from build123d import *

# Parameters (mm, degrees)
SKETCH1_R           = 4.9609375
BOSS_EXTRUDE1_DEPTH = 75.692
SKETCH3_R           = 1.6256
CUT_EXTRUDE1_DEPTH  = 11.914472708
SKETCH3_3_R         = 2.511415146
SKETCH3_3_R_2       = 1.6256
BOSS_EXTRUDE2_DEPTH = 5.08
SKETCH4_R           = 1.580559699
SKETCH4_R_2         = 1.615968851
SKETCH4_R_3         = 1.651
CUT_EXTRUDE2_DEPTH  = 11.914472708
BOSS_EXTRUDE3_DEPTH = 5.500116
SKETCH6_R           = 1.5875
CUT_EXTRUDE3_DEPTH  = 17.414588708


with BuildPart() as part:
    # Sketch1 → Boss-Extrude1 (new body, symmetric)
    with BuildSketch(Plane(origin=(0, 0, 0), x_dir=(1, 0, 0), z_dir=(0, 1, 0))):
        with BuildLine():
            ThreePointArc((-54.898232946, 10.914472708), (-55.979756859, 9.486084273), (-57.024125462, 8.030308975))
            ThreePointArc((-57.024125462, 8.030308975), (-55.271492218, -9.123122127), (-40.64, 0))
            Line((-40.64, 0), (40.64, 0))
            ThreePointArc((40.64, 0), (55.271492218, -9.123122127), (57.024125462, 8.030308975))
            ThreePointArc((57.024125462, 8.030308975), (55.979756859, 9.486084273), (54.898232946, 10.914472708))
            Line((54.898232946, 10.914472708), (-54.898232946, 10.914472708))
        make_face()
        with Locations((-50.8, 0)):
            Circle(SKETCH1_R, mode=Mode.SUBTRACT)
        with Locations((50.8, 0)):
            Circle(SKETCH1_R, mode=Mode.SUBTRACT)
    extrude(amount=BOSS_EXTRUDE1_DEPTH, both=True)

    # Sketch3 → Cut-Extrude1 (cut, through all)
    with BuildSketch(Plane.XY):
        with Locations((-14.08707582, 68.405041605)):
            Circle(SKETCH3_R)
        with Locations((-26.78707582, 43.005041605)):
            Circle(SKETCH3_R)
    extrude(amount=-CUT_EXTRUDE1_DEPTH, mode=Mode.SUBTRACT)

    # Sketch3_3 → Boss-Extrude2 (add)
    with BuildSketch(Plane.XY):
        with Locations((-14.08707582, 68.405041605)):
            Circle(SKETCH3_3_R)
        with Locations((-14.08707582, 68.405041605)):
            Circle(SKETCH3_3_R_2, mode=Mode.SUBTRACT)
        with Locations((-26.78707582, 43.005041605)):
            Circle(SKETCH3_3_R)
        with Locations((-26.78707582, 43.005041605)):
            Circle(SKETCH3_3_R_2, mode=Mode.SUBTRACT)
    extrude(amount=BOSS_EXTRUDE2_DEPTH)

    # Sketch4 → Cut-Extrude2 (cut, through all)
    with BuildSketch(Plane.XY):
        with Locations((5.097142458, 69.338036856)):
            Circle(SKETCH4_R)
        with Locations((27.569466172, 69.326708036)):
            Circle(SKETCH4_R_2)
        with Locations((4.630258258, 15.178805596)):
            Circle(SKETCH4_R_3)
        with Locations((31.55425332, 15.195112998)):
            Circle(SKETCH4_R_3)
    extrude(amount=-CUT_EXTRUDE2_DEPTH, mode=Mode.SUBTRACT)

    # Sketch5 → Boss-Extrude3 (add)
    with BuildSketch(Plane.XY):
        Polygon((-32.457787853, 17.360692428), (-24.837787853, 17.360692428), (-24.837787853, 23.710692428), (-38.807787853, 23.710692428), (-38.807787853, -27.089307572), (-0.707787853, -27.089307572), (-0.707787853, 23.710692428), (-14.677787853, 23.710692428), (-14.677787853, 17.360692428), (-7.057787853, 17.360692428), (-7.057787853, -20.739307572), (-32.457787853, -20.739307572), align=None)
    extrude(amount=BOSS_EXTRUDE3_DEPTH)

    # Sketch6 → Cut-Extrude3 (cut, through all)
    with BuildSketch(Plane.XY.offset(5.500116)):
        with Locations((-35.482909848, 20.385814423)):
            Circle(SKETCH6_R)
        with Locations((-4.032665858, -23.764429567)):
            Circle(SKETCH6_R)
    extrude(amount=-CUT_EXTRUDE3_DEPTH, mode=Mode.SUBTRACT)


solid = part.part
Geometry: final body of the model. Coordinates: model frame, mm. A direction names the side the tool comes from. Round coordinates to 2 decimals unless told otherwise and drop trailing zeros. Loops run counter-clockwise (first coordinate to the right, second up) from the corner with the lowest first, then second, coordinate; pieces in that order, holes last. Notation, with made-up numbers: (-1.5, 56) -> (29.5, 56) arc R9 ccw to (29.5, 73) -> close; hole circle Ø5 at (-35, 83). An arc over 180 degrees is marked (long way). One line per question, with ' | ' between items. Start each with the question number.
1. Mould query, pull axis Y, two halves, no side actions, for faces 1 (the face through (-55.756, -1.06, -0.218)), 2 (the face through (-20, -20.739, 3)), 3 (the face through (27.36, 70.93, -5.38)). Classes: pulls with the +Y half, pulls with the -Y half, needs draft (parallel to the pull), parting line crosses it, or undercut.
2. Contact query for flat-ended pins moving along their axis: pin 1 (5.5 mm diameter, centred on x = -13.5, y = 68, fed in from +Z); pin 2 (3 mm diameter, centred on y = -2, z = 4, fed in from +X); pin 3 (1.7 mm diameter, centred on y = -1, z = 3, fed in from -X). Output: stop coordinate, or through.
3. Line query: line 1 along X through (y, z) = (12, -0.25); line 2 along Z through (x, y) = (51, -39.5); line 3 along X through (y, z) = (2, 1.75). Output: solid intervals per line, ascending. Write a range as [from, to].
4. Section B-B on x = 50.8. Output: boundary loops of the cut face in (y, z), and give its area (3 significant figures).
5. Section D-D on y = -56. Output: boundary loops of the cut face in (x, z), and give its area (3 significant figures).
6. Set-up query: faces 4 (the face through (-38.808, -1, 3)), 5 (the face through (-11, 17.361, 3)), 6 (the face through (55.011, 1.06, 9.246)), 7 (the face through (-25, 43, 5.08)). Return all of +Z, -Z, +X, -X, +Y, -Y with unobstructed straight access to the full face (end or side cutting, diameter ignored); none if empty.
7. Section A-A on y = -3. Output: boundary loops of the cut face in (x, z).
8. Section C-C on z = 3. Count the separate pieces of the cut face and the enclosed holes in it, and give its area (3 significant figures).
Returned:
1) face 1: needs draft | face 2: undercut | face 3: undercut
2) pin 1: stops at z = 5.08 | pin 2: stops at x = 60.65 | pin 3: stops at x = -60.73
3) line 1: x = [-60.96, -55.75], [-45.85, 45.85], [55.75, 60.96] | line 2: z = [-10.91, -4.96], [4.96, 10.16] | line 3: x = [-60.81, -55.44], [-46.16, -40.79], [-38.81, -32.46], [-7.06, -0.71], [40.79, 46.16], [55.44, 60.81]
4) outline: (-75.69, -10.91) -> (75.69, -10.91) -> (75.69, -4.96) -> (-75.69, -4.96) -> close; (-75.69, 4.96) -> (75.69, 4.96) -> (75.69, 10.16) -> (-75.69, 10.16) -> close | area: 1,690 mm2
5) outline: (-57.02, -8.03) arc R69.54 ccw to (-54.9, -10.91) -> (54.9, -10.91) arc R69.54 ccw to (57.02, -8.03) arc R10.16 ccw (long way) to (40.64, 0) -> (-40.64, 0) arc R10.16 ccw (long way) to start; hole circle Ø9.92 at (-50.8, 0); hole circle Ø9.92 at (50.8, 0) | area: 1,450 mm2
6) face 4: +Z, +Y, -Y | face 5: +Z | face 6: +Y, -Y | face 7: +Z, +Y
7) outline: (-57.02, -8.03) arc R69.54 ccw to (-54.9, -10.91) -> (54.9, -10.91) arc R69.54 ccw to (57.02, -8.03) arc R10.16 ccw (long way) to (40.64, 0) -> (-0.71, 0) -> (-0.71, 5.5) -> (-7.06, 5.5) -> (-7.06, 0) -> (-32.46, 0) -> (-32.46, 5.5) -> (-38.81, 5.5) -> (-38.81, 0) -> (-40.64, 0) arc R10.16 ccw (long way) to start; hole circle Ø9.92 at (-50.8, 0); hole circle Ø9.92 at (50.8, 0)
8) separate pieces: 7 | enclosed holes: 4 | area: 4,400 mm2
